```python
from build123d import *

# Parameters (mm, degrees)
EXTRUDE_1_DEPTH   = 6.5
EXTRUDE_1_2_DEPTH = 6.5
SKETCH_1_3_R      = 2
EXTRUDE_2_DEPTH   = 25
SKETCH_1_4_R      = 2
EXTRUDE_3_DEPTH   = 3
SKETCH_1_13_R     = 1.25
EXTRUDE_8_DEPTH   = 7.5
SKETCH_1_12_R     = 1.25
EXTRUDE_7_DEPTH   = 7.5


with BuildPart() as part:
    # Sketch 1 → Extrude 1 (new body)
    with BuildSketch(Plane(origin=(0, 0, 0), x_dir=(1, 0, 0), z_dir=(0, 1, 0))):
        with BuildLine():
            ThreePointArc((-32, 23), (-31.089439395, 26.177673149), (-28.63413112, 28.390858303))
            Line((-28.63413112, 28.390858303), (-45.533328715, 20.133415836))
            ThreePointArc((-45.533328715, 20.133415836), (-46.601585329, 19.210972795), (-47, 17.856964263))
            Line((-47, 17.856964263), (-47, -17.856964263))
            ThreePointArc((-47, -17.856964263), (-46.601585329, -19.210972795), (-45.533328715, -20.133415836))
            Line((-45.533328715, -20.133415836), (-28.63413112, -28.390858303))
            ThreePointArc((-28.63413112, -28.390858303), (-31.089439395, -26.177673149), (-32, -23))
            Line((-32, -23), (-32, 23))
        make_face()
        with BuildLine():
            Line((-41.5, -7.5), (-41.5, -3.75))
            ThreePointArc((-41.5, -3.75), (-43.75, 0), (-41.5, 3.75))
            Line((-41.5, 3.75), (-41.5, 7.5))
            ThreePointArc((-41.5, 7.5), (-39.5, 9.5), (-37.5, 7.5))
            Line((-37.5, 7.5), (-37.5, 3.75))
            ThreePointArc((-37.5, 3.75), (-35.25, 0), (-37.5, -3.75))
            Line((-37.5, -3.75), (-37.5, -7.5))
            ThreePointArc((-37.5, -7.5), (-39.5, -9.5), (-41.5, -7.5))
        make_face(mode=Mode.SUBTRACT)
    extrude(amount=EXTRUDE_1_DEPTH)



with BuildPart() as body_2:
    # Sketch 1 → Extrude 1 2 (new body)
    with BuildSketch(Plane(origin=(0, 0, 0), x_dir=(1, 0, 0), z_dir=(0, 1, 0))):
        with BuildLine():
            Line((45.533328715, 20.133415836), (28.63413112, 28.390858303))
            ThreePointArc((28.63413112, 28.390858303), (31.089439395, 26.177673149), (32, 23))
            Line((32, 23), (32, -23))
            ThreePointArc((32, -23), (31.089439395, -26.177673149), (28.63413112, -28.390858303))
            Line((28.63413112, -28.390858303), (45.533328715, -20.133415836))
            ThreePointArc((45.533328715, -20.133415836), (46.601585329, -19.210972795), (47, -17.856964263))
            Line((47, -17.856964263), (47, 17.856964263))
            ThreePointArc((47, 17.856964263), (46.601585329, 19.210972795), (45.533328715, 20.133415836))
        make_face()
        with BuildLine():
            Line((37.5, -7.5), (37.5, -3.75))
            ThreePointArc((37.5, -3.75), (35.25, 0), (37.5, 3.75))
            Line((37.5, 3.75), (37.5, 7.5))
            ThreePointArc((37.5, 7.5), (39.5, 9.5), (41.5, 7.5))
            Line((41.5, 7.5), (41.5, 3.75))
            ThreePointArc((41.5, 3.75), (43.75, 0), (41.5, -3.75))
            Line((41.5, -3.75), (41.5, -7.5))
            ThreePointArc((41.5, -7.5), (39.5, -9.5), (37.5, -7.5))
        make_face(mode=Mode.SUBTRACT)
    extrude(amount=EXTRUDE_1_2_DEPTH)


with BuildPart() as part_1:
    add(part.part)

    add(body_2.part)  # Extrude 2 merges body 2
    # Sketch 1_3 → Extrude 2 (add)
    with BuildSketch(Plane(origin=(0, 0, 0), x_dir=(1, 0, 0), z_dir=(0, 1, 0))):
        with BuildLine():
            ThreePointArc((-26, -29), (-30.242640687, -27.242640687), (-32, -23))
            Line((-32, -23), (-32, 23))
            ThreePointArc((-32, 23), (-30.242640687, 27.242640687), (-26, 29))
            Line((-26, 29), (26, 29))
            ThreePointArc((26, 29), (30.242640687, 27.242640687), (32, 23))
            Line((32, 23), (32, -23))
            ThreePointArc((32, -23), (30.242640687, -27.242640687), (26, -29))
            Line((26, -29), (-26, -29))
        make_face()
        with Locations(Location((-26, -23, 0), (0, 0, 270))):
            Circle(SKETCH_1_3_R, mode=Mode.SUBTRACT)
        with Locations(Location((26, -23, 0), (0, 0, 270))):
            Circle(SKETCH_1_3_R, mode=Mode.SUBTRACT)
        with Locations(Location((-26, 23, 0), (0, 0, 270))):
            Circle(SKETCH_1_3_R, mode=Mode.SUBTRACT)
        with Locations(Location((26, 23, 0), (0, 0, 270))):
            Circle(SKETCH_1_3_R, mode=Mode.SUBTRACT)
        with BuildLine():
            ThreePointArc((-12.75, -23), (-13.99479618, -19.99479618), (-17, -18.75))
            Line((-17, -18.75), (-23.366086562, -18.75))
            ThreePointArc((-23.366086562, -18.75), (-21.020896599, -22.543349889), (-22.636965656, -26.7))
            Line((-22.636965656, -26.7), (-11.113034344, -26.7))
            ThreePointArc((-11.113034344, -26.7), (-12.322481368, -25.022971611), (-12.75, -23))
        make_face(mode=Mode.SUBTRACT)
        with BuildLine():
            ThreePointArc((-10.75, -23), (-9.871320344, -25.121320344), (-7.75, -26))
            Line((-7.75, -26), (16.75, -26))
            ThreePointArc((16.75, -26), (18.871320344, -25.121320344), (19.75, -23))
            ThreePointArc((19.75, -23), (21.580582618, -18.580582618), (26, -16.75))
            ThreePointArc((26, -16.75), (28.121320344, -15.871320344), (29, -13.75))
            Line((29, -13.75), (29, 13.75))
            ThreePointArc((29, 13.75), (28.121320344, 15.871320344), (26, 16.75))
            Line((26, 16.75), (17, 16.75))
            ThreePointArc((17, 16.75), (12.580582618, 18.580582618), (10.75, 23))
            ThreePointArc((10.75, 23), (9.871320344, 25.121320344), (7.75, 26))
            Line((7.75, 26), (-16.75, 26))
            ThreePointArc((-16.75, 26), (-18.871320344, 25.121320344), (-19.75, 23))
            ThreePointArc((-19.75, 23), (-21.580582618, 18.580582618), (-26, 16.75))
            ThreePointArc((-26, 16.75), (-28.121320344, 15.871320344), (-29, 13.75))
            Line((-29, 13.75), (-29, -13.75))
            ThreePointArc((-29, -13.75), (-28.121320344, -15.871320344), (-26, -16.75))
            Line((-26, -16.75), (-17, -16.75))
            ThreePointArc((-17, -16.75), (-12.580582618, -18.580582618), (-10.75, -23))
        make_face(mode=Mode.SUBTRACT)
        with BuildLine():
            ThreePointArc((12.75, 23), (13.99479618, 19.99479618), (17, 18.75))
            Line((17, 18.75), (23.366086562, 18.75))
            ThreePointArc((23.366086562, 18.75), (21.020896599, 22.543349889), (22.636965656, 26.7))
            Line((22.636965656, 26.7), (11.113034344, 26.7))
            ThreePointArc((11.113034344, 26.7), (12.322481368, 25.022971611), (12.75, 23))
        make_face(mode=Mode.SUBTRACT)
    extrude(amount=EXTRUDE_2_DEPTH)

    # Sketch 1_4 → Extrude 3 (add)
    with BuildSketch(Plane(origin=(0, 0, 0), x_dir=(1, 0, 0), z_dir=(0, 1, 0))):
        with BuildLine():
            ThreePointArc((10.75, 23), (9.871320344, 25.121320344), (7.75, 26))
            Line((7.75, 26), (-16.75, 26))
            ThreePointArc((-16.75, 26), (-18.871320344, 25.121320344), (-19.75, 23))
            ThreePointArc((-19.75, 23), (-21.580582618, 18.580582618), (-26, 16.75))
            ThreePointArc((-26, 16.75), (-28.121320344, 15.871320344), (-29, 13.75))
            Line((-29, 13.75), (-29, -13.75))
            ThreePointArc((-29, -13.75), (-28.121320344, -15.871320344), (-26, -16.75))
            Line((-26, -16.75), (-17, -16.75))
            ThreePointArc((-17, -16.75), (-12.580582618, -18.580582618), (-10.75, -23))
            ThreePointArc((-10.75, -23), (-9.871320344, -25.121320344), (-7.75, -26))
            Line((-7.75, -26), (16.75, -26))
            ThreePointArc((16.75, -26), (18.871320344, -25.121320344), (19.75, -23))
            ThreePointArc((19.75, -23), (21.580582618, -18.580582618), (26, -16.75))
            ThreePointArc((26, -16.75), (28.121320344, -15.871320344), (29, -13.75))
            Line((29, -13.75), (29, 13.75))
            ThreePointArc((29, 13.75), (28.121320344, 15.871320344), (26, 16.75))
            Line((26, 16.75), (17, 16.75))
            ThreePointArc((17, 16.75), (12.580582618, 18.580582618), (10.75, 23))
        make_face()
        with BuildLine():
            ThreePointArc((12.75, 23), (13.99479618, 19.99479618), (17, 18.75))
            Line((17, 18.75), (23.366086562, 18.75))
            ThreePointArc((23.366086562, 18.75), (21.020896599, 22.543349889), (22.636965656, 26.7))
            Line((22.636965656, 26.7), (11.113034344, 26.7))
            ThreePointArc((11.113034344, 26.7), (12.322481368, 25.022971611), (12.75, 23))
        make_face()
        with BuildLine():
            ThreePointArc((-23.366086562, -18.75), (-21.020896599, -22.543349889), (-22.636965656, -26.7))
            Line((-22.636965656, -26.7), (-11.113034344, -26.7))
            ThreePointArc((-11.113034344, -26.7), (-12.322481368, -25.022971611), (-12.75, -23))
            ThreePointArc((-12.75, -23), (-13.99479618, -19.99479618), (-17, -18.75))
            Line((-17, -18.75), (-23.366086562, -18.75))
        make_face()
        with Locations(Location((-26, 23, 0), (0, 0, 270))):
            Circle(SKETCH_1_4_R)
        with Locations(Location((26, 23, 0), (0, 0, 270))):
            Circle(SKETCH_1_4_R)
        with Locations(Location((26, -23, 0), (0, 0, 270))):
            Circle(SKETCH_1_4_R)
        with Locations(Location((-26, -23, 0), (0, 0, 270))):
            Circle(SKETCH_1_4_R)
    extrude(amount=EXTRUDE_3_DEPTH)

    # Sketch 1_13 → Extrude 8 (add)
    # profile 1 of 2: a face of its own
    with BuildSketch(Plane(origin=(0, 0, 0), x_dir=(1, 0, 0), z_dir=(0, 1, 0))):
        with BuildLine():
            Line((-11.5, 1.322875656), (-11.5, 6.01))
            ThreePointArc((-11.5, 6.01), (-11.063589104, 7.063589104), (-10.01, 7.5))
            Line((-10.01, 7.5), (-9.99, 7.5))
            ThreePointArc((-9.99, 7.5), (-8.936410896, 7.063589104), (-8.5, 6.01))
            Line((-8.5, 6.01), (-8.5, 1.322875656))
            ThreePointArc((-8.5, 1.322875656), (-8, 0), (-8.5, -1.322875656))
            Line((-8.5, -1.322875656), (-8.5, -6.01))
            ThreePointArc((-8.5, -6.01), (-8.936410896, -7.063589104), (-9.99, -7.5))
            Line((-9.99, -7.5), (-10.01, -7.5))
            ThreePointArc((-10.01, -7.5), (-11.063589104, -7.063589104), (-11.5, -6.01))
            Line((-11.5, -6.01), (-11.5, -1.322875656))
            ThreePointArc((-11.5, -1.322875656), (-12, 0), (-11.5, 1.322875656))
        make_face()
        with Locations(Location((-10, 0, 0), (0, 0, 270))):
            Circle(SKETCH_1_13_R, mode=Mode.SUBTRACT)
    # profile 2 of 2: a face of its own
    with BuildSketch(Plane(origin=(0, 0, 0), x_dir=(1, 0, 0), z_dir=(0, 1, 0))):
        with BuildLine():
            Line((8.5, -6.01), (8.5, -1.322875656))
            ThreePointArc((8.5, -1.322875656), (8, 0), (8.5, 1.322875656))
            Line((8.5, 1.322875656), (8.5, 6.01))
            ThreePointArc((8.5, 6.01), (8.936410896, 7.063589104), (9.99, 7.5))
            Line((9.99, 7.5), (10.01, 7.5))
            ThreePointArc((10.01, 7.5), (11.063589104, 7.063589104), (11.5, 6.01))
            Line((11.5, 6.01), (11.5, 1.322875656))
            ThreePointArc((11.5, 1.322875656), (12, 0), (11.5, -1.322875656))
            Line((11.5, -1.322875656), (11.5, -6.01))
            ThreePointArc((11.5, -6.01), (11.063589104, -7.063589104), (10.01, -7.5))
            Line((10.01, -7.5), (9.99, -7.5))
            ThreePointArc((9.99, -7.5), (8.936410896, -7.063589104), (8.5, -6.01))
        make_face()
        with Locations(Location((10, 0, 0), (0, 0, 90))):
            Circle(SKETCH_1_13_R, mode=Mode.SUBTRACT)
    extrude(amount=EXTRUDE_8_DEPTH)

    # Sketch 1_12 → Extrude 7 (add)
    # profile 1 of 2: a face of its own
    with BuildSketch(Plane(origin=(0, 0, 0), x_dir=(1, 0, 0), z_dir=(0, 1, 0))):
        with BuildLine():
            Line((-8.5, -6.01), (-8.5, -1.322875656))
            ThreePointArc((-8.5, -1.322875656), (-8, 0), (-8.5, 1.322875656))
            Line((-8.5, 1.322875656), (-8.5, 6.01))
            ThreePointArc((-8.5, 6.01), (-8.936410896, 7.063589104), (-9.99, 7.5))
            Line((-9.99, 7.5), (-10.01, 7.5))
            ThreePointArc((-10.01, 7.5), (-11.063589104, 7.063589104), (-11.5, 6.01))
            Line((-11.5, 6.01), (-11.5, 1.322875656))
            ThreePointArc((-11.5, 1.322875656), (-12, 0), (-11.5, -1.322875656))
            Line((-11.5, -1.322875656), (-11.5, -6.01))
            ThreePointArc((-11.5, -6.01), (-11.063589104, -7.063589104), (-10.01, -7.5))
            Line((-10.01, -7.5), (-9.99, -7.5))
            ThreePointArc((-9.99, -7.5), (-8.936410896, -7.063589104), (-8.5, -6.01))
        make_face()
        with Locations(Location((-10, 0, 0), (0, 0, 270))):
            Circle(SKETCH_1_12_R, mode=Mode.SUBTRACT)
    # profile 2 of 2: a face of its own
    with BuildSketch(Plane(origin=(0, 0, 0), x_dir=(1, 0, 0), z_dir=(0, 1, 0))):
        with BuildLine():
            ThreePointArc((11.5, 1.322875656), (12, 0), (11.5, -1.322875656))
            Line((11.5, -1.322875656), (11.5, -6.01))
            ThreePointArc((11.5, -6.01), (11.063589104, -7.063589104), (10.01, -7.5))
            Line((10.01, -7.5), (9.99, -7.5))
            ThreePointArc((9.99, -7.5), (8.936410896, -7.063589104), (8.5, -6.01))
            Line((8.5, -6.01), (8.5, -1.322875656))
            ThreePointArc((8.5, -1.322875656), (8, 0), (8.5, 1.322875656))
            Line((8.5, 1.322875656), (8.5, 6.01))
            ThreePointArc((8.5, 6.01), (8.936410896, 7.063589104), (9.99, 7.5))
            Line((9.99, 7.5), (10.01, 7.5))
            ThreePointArc((10.01, 7.5), (11.063589104, 7.063589104), (11.5, 6.01))
            Line((11.5, 6.01), (11.5, 1.322875656))
        make_face()
        with Locations(Location((10, 0, 0), (0, 0, 90))):
            Circle(SKETCH_1_12_R, mode=Mode.SUBTRACT)
    extrude(amount=EXTRUDE_7_DEPTH)


solid = part_1.part
```
Read the model definition and answer for the solid it produces. Units are mm, in the model's axes. A direction names the side the tool comes from. Give positions to 0.01 mm unless a question says otherwise; leave off trailing zeros. Loops run counter-clockwise (first coordinate to the right, second up) from the corner with the lowest first, then second, coordinate; pieces in that order, holes last.
Item 1: The part is cut by section A-A (z = -5). Write down the section's boundary in (x, y), and give its area (3 significant figures).
Item 2: The part is cut by section B-B (x = 39.5). Write down the section's boundary in (y, z).
Item 3: The part is cut by section C-C (z = 11). Write down the section's boundary in (x, y).
Item 4: The mould has two halves that part along Z. Classify faces 4 (the flat face through (1, 0, 0)), 5 (the cylindrical face through (24, 14, -23)), 6 (the cylindrical face through (46.612, 3.204, -19.194)), 7 (the flat face through (36.965, 3.204, 24.32)): released by +Z, released by -Z, zero draft, split by the parting line, or undercut.
Item 5: The part is cut by section D-D (y = 20.5). Give the number of separate pieces and of enclosed holes in the cut face, and give its area (3 significant figures).
Item 6: Find the intervals of material crossed by line 1 along X through (y, z) = (15.25, -23); line 2 along X through (y, z) = (17.5, 23); line 3 along Z through (x, y) = (10, 5.35), in increasing order.
Item 7: Each of these flat-tipped pins is pushed along its axis until it touches: pin 1 Ø4.5 at (x, z) = (-26, -23) entering from -Y; pin 2 Ø3 at (x, z) = (13, 19) entering from +Y; pin 3 Ø5 at (x, z) = (7, -7.5) entering from +Y; pin 4 Ø1 at (y, z) = (12.5, -2.5) entering from -X. Where does it stop, or does it pass through?
Item 8: For faces 1 (the cylindrical face through (30.289, 15.103, 27.196)), 2 (the flat face through (11.5, 5, 4)), 3 (the cylindrical face through (-39.5, 3.2, 9.5)), determine the directions among +Z, -Z, +X, -X, +Y, -Y from which every point of the face is accessible in a straight line to the end or side of a thin tool.
Taken from the geometry:
1. outline: (-47, 0) - (-41.5, 0) - (-41.5, 6.5) - (-47, 6.5) - close; (-37.5, 0) - (37.5, 0) - (37.5, 6.5) - (32, 6.5) - (32, 25) - (29, 25) - (29, 3) - (11.5, 3) - (11.5, 7.5) - (8.5, 7.5) - (8.5, 3) - (-8.5, 3) - (-8.5, 7.5) - (-11.5, 7.5) - (-11.5, 3) - (-29, 3) - (-29, 25) - (-32, 25) - (-32, 6.5) - (-37.5, 6.5) - close; (41.5, 0) - (47, 0) - (47, 6.5) - (41.5, 6.5) - close
1. area: 494 mm2
2. outline: (0, -23.08) - (6.5, -23.08) - (6.5, -9.5) - (0, -9.5) - close; (0, 9.5) - (6.5, 9.5) - (6.5, 23.08) - (0, 23.08) - close
3. outline: (-47, 0) - (47, 0) - (47, 6.5) - (32, 6.5) - (32, 25) - (29, 25) - (29, 3) - (-29, 3) - (-29, 25) - (-32, 25) - (-32, 6.5) - (-47, 6.5) - close
4. face 4: zero draft
4. face 5: undercut
4. face 6: released by -Z
4. face 7: released by +Z
5. separate pieces: 1
5. enclosed holes: 7
5. area: 969 mm2
6. line 1: x = -32 to -28, -24 to -19.75, 10.75 to 12.75, 21 to 24, 28 to 32
6. line 2: x = -32 to -28, -24 to -21, -12.75 to -10.75, 19.75 to 24, 28 to 32
6. line 3: z = -29 to -24.98, -7.5 to -1.25, 1.25 to 7.5, 26 to 29
7. pin 1: stops at y = 0
7. pin 2: stops at y = 3
7. pin 3: stops at y = 7.5
7. pin 4: stops at x = -32
8. face 1: +Z, +X, +Y
8. face 2: +Y
8. face 3: +Y, -Y
